Model file for the job. Use its own axes, mm. A direction names the side the tool comes from. Coordinates: 2 decimals unless noted, no trailing zeros. Order: outer loops, then holes, each group sorted by start corner. A loop starts at its lowest first (then second) coordinate and runs counter-clockwise, first axis right, second up. Notation, with made-up numbers: (-24.75, 18) -> (-3.75, 18) arc R20 ccw to (-3.75, 46) -> close; hole circle Ø9 at (-26, -4.75). An arc over 180 degrees is marked (long way). Return JSON: item names as keys, results as strings. Group by question number.
1) Pull direction X, two halves, no side cores. Call faces 3 (the flat face through (-12.8, -40.2, 4.6)), 4 (the flat face through (-75, 51.4, 4.9)), 5 (the flat face through (60, 48.6, 4.9)), 6 (the flat face through (-22, 49, 10)): +X half, -X half, draft (parallel to the pull), parting line (faces both ways), or undercut.
2) Cut at D-D (y = 99.5). Write the cut outline in (x, z).
3) Which spindle directions (+Z, -Z, +X, -X, +Y, -Y) get a long thin tool onto all of the face, cutting with end or side? Do faces 1 (the cylindrical face through (33.763, 135.902, 7.042)), 2 (the flat face through (-7, -50, 5)). Say none if no direction does.
4) Probe line 1 (X direction, y = 65, z = 3.5); line 2 (Y direction, x = 53.25, z = 5); line 3 (Z direction, x = 54.25, y = 125). List the from-to ranges inside material, lowest first.
5) Cut at C-C (z = 1.75). State how many separate pieces and enclosed holes the cut face has, and give its area (3 significant figures).
6) Cut at B-B (x = -30). Write the cut outline in (y, z), and give its area (3 significant figures).
7) Cut at A-A (y = -38). Write the cut outline in (x, z), and give its area (3 significant figures).
8) Flat gauge pin, fed straight in: pin 1 (8.5 mm diameter, centred on x = 30, y = 0, fed in from +Z). Where does the tip first touch, or does it go through?
Autodesk Inventor part; units mm, degrees
ref_plane "Arbeitsebene1" through (-7.5, -50, 10) normal (1, 0, 0) x (0, 0, -1)
ref_plane "YZ Plane" through (0, 0, 0) normal (1, 0, 0) x (0, 1, 0)
ref_plane "XZ Plane" through (0, 0, 0) normal (0, 1, 0) x (-1, 0, 0)
sketch "Skizze1" plane through (0, 0, 0) normal (0, 0, 1) x (1, 0, 0)
  line L0 (-60, 110) -> (60, 110)
  line L1 (60, 110) -> (60, -50)
  line L2 (60, -50) -> (-60, -50)
  line L3 (-60, -50) -> (-60, 110)
  line L4 (-1104, 0) -> (254, 0)
  line L5 (0, -83) -> (0, 148)
  circle A0 centre (-30, 0) radius 2.7
  circle A1 centre (30, 0) radius 2.7
  line L6 (-910, 115) -> (-40, 115)
  point P0 (0, 0)
  dimension "d0" = 110
  dimension "d1" = 120
  dimension "d2" = 60
  dimension "d3" = 5.4
  dimension "d7" = 50
extrude "Extrusion1" add sketch "Skizze1" along normal blind 10 contours L0 L5 L4 A0 L3 | L0 L1 L4 A1 L5 | L4 A0 L5 L2 L3 | L4 A1 L1 L2 L5
sketch "Skizze2" plane through (0, 0, 10) normal (0, 0, 1) x (1, 0, 0)
  line L0 (-60, 110) -> (60, 110)
  line L1 (0, -82) -> (0, 142)
  point P0 (0, 0)
  point P1 (0, 90)
  point P2 (0, 40)
  dimension "d17" = 20
  dimension "d18" = 50
hole "Bohrung2" at (0, 90, 10) at (0, 40, 10) direction (0, 0, -1) diameter 34 end through all
sketch "Skizze5" plane through (0, 0, 10) normal (0, 0, 1) x (1, 0, 0)
  circle A0 centre (30, 0) radius 2.7
  circle A1 centre (-30, 0) radius 2.7
  circle A2 centre (-30, 0) radius 7
  circle A3 centre (30, 0) radius 7
  point P0 (0, 0)
  dimension "d33" = 14
extrude "Extrusion2" cut sketch "Skizze5" against normal blind 6
sketch "Skizze6" plane through (-60, 110, 0) normal (0, 1, 0) x (1, 0, 0)
  line L0 (0, -10) -> (120, -10)
  line L1 (120, 0) -> (120, -10)
  line L2 (0, 0) -> (120, 0)
  line L3 (0, 0) -> (0, -10)
  point P0 (60, 0)
extrude "Extrusion3" add sketch "Skizze6" along normal blind 40
pattern_linear "Rechteckige Anordnung1" count 2 spacing 130 along (0, 1, 0) of "Extrusion2"
sketch "Skizze8" plane through (0, 0, 10) normal (0, 0, 1) x (1, 0, 0)
  circle A0 centre (30, 130) radius 7
  circle A1 centre (-30, 130) radius 7
  point P0 (0, 0)
hole "Bohrung4" at (-30, 130, 10) at (30, 130, 10) direction (0, 0, -1) diameter 5.4 end through all
sketch "Skizze9" plane through (-60, -50, 0) normal (-1, 0, 0) x (0, 0, 1)
  line L0 (10, 0) -> (10, 200)
  line L1 (10, 200) -> (0, 200)
  line L2 (0, 0) -> (0, 200)
  line L3 (0, 0) -> (10, 0)
  point P0 (0, 50)
extrude "Extrusion4" add sketch "Skizze9" along normal blind 15
sketch "Skizze10" plane through (0, 0, 10) normal (0, 0, 1) x (1, 0, 0)
  line L0 (60, 150) -> (-75, 150)
  line L1 (-75, 150) -> (-75, -50)
  line L2 (60, -50) -> (-75, -50)
  line L3 (-75, 120) -> (-28.668, 120)
  line L4 (-53, 93.8234) -> (-53, 98.8806)
  line L5 (60, 150) -> (60, -50)
  line L6 (-75, 10) -> (-27.5048, 10)
  point P0 (0, 0)
  point P1 (-62, 120)
  point P2 (-44, 120)
  point P3 (-62, 10)
  point P4 (-44, 10)
  dimension "d50" = 30
  dimension "d51" = 22
  dimension "d52" = 18
  dimension "d60" = 140
  dimension "d61" = 18
hole "Bohrung6" at (-62, 120, 10) at (-44, 120, 10) at (-62, 10, 10) at (-44, 10, 10) direction (0, 0, -1) diameter 3.242 end through all
sketch "Skizze11" plane through (0, 0, 10) normal (0, 0, 1) x (1, 0, 0)
  circle A0 centre (7.5, -46) radius 1.621
  circle A1 centre (7.5, -30) radius 1.621
  circle A2 centre (-7.5, -30) radius 1.621
  circle A3 centre (-7.5, -46) radius 1.621
  line L0 (-25, -26) -> (25, -26)
  line L1 (-25, -50) -> (-25, -26)
  line L2 (25, -50) -> (-25, -50)
  line L3 (25, -26) -> (25, -50)
  line L4 (-25, -38) -> (25, -38)
  line L5 (-102, 0) -> (87, 0)
  line L6 (0, -90) -> (0, 190)
  circle A4 centre (15, -38) radius 2.067
  circle A5 centre (-15, -38) radius 2.067
  point P0 (0, 0)
  point P1 (-15, -38)
  point P2 (15, -38)
  dimension "d69" = 30
hole "Bohrung7" at (-15, -38, 10) at (15, -38, 10) direction (0, 0, -1) diameter 5.5 end through all counterbore diameter 10 counterbore depth 5.4
sketch "Skizze12" plane through (60, -50, 10) normal (1, 0, 0) x (0, 0, -1)
  line L0 (0, 200) -> (0, 0)
  line L1 (10, 0) -> (0, 0)
  line L2 (10, 200) -> (0, 200)
  line L3 (10, -40) -> (10, 240)
  line L4 (12, 50) -> (-2, 50)
  line L5 (0, 100) -> (10, 100)
  line L6 (5, 200) -> (5, 0)
  point P0 (10, 50)
  point P1 (5, 175)
  point P2 (5, 100)
  point P3 (5, 25)
  dimension "d77" = 25
  dimension "d78" = 25
hole "Bohrung8" at (60, 125, 5) at (60, 50, 5) at (60, -25, 5) direction (-1, 0, 0) diameter 2.459 depth 10 tip angle 118
ref_plane "Arbeitsebene1" through (-7.5, -50, 10) normal (1, 0, 0) x (0, 0, -1)
mirror "Spiegeln1" about plane through (-7.5, -50, 10) normal (1, 0, 0) of "Bohrung8"
hole "Bohrung9" at (8, 65, 10) at (-8, 65, 10) direction (0, 0, -1) diameter 5 end through all
sketch "Skizze13" plane through (0, 0, 10) normal (0, 0, 1) x (1, 0, 0)
  circle A0 centre (-15, 119) radius 2.75
  circle A1 centre (15, 119) radius 2.75
  circle A2 centre (15, 11) radius 2.75
  circle A3 centre (-15, 11) radius 2.75
  point P0 (0, 0)
hole "Bohrung10" at (-15, 11, 10) at (15, 11, 10) at (15, 119, 10) at (-15, 119, 10) direction (0, 0, -1) diameter 4.134 end through all
sketch "Skizze14" plane through (0, 0, 10) normal (0, 0, 1) x (1, 0, 0)
  line L0 (60, 150) -> (60, -50)
  line L1 (60, 150) -> (-75, 150)
  line L2 (-75, 150) -> (-75, -50)
  line L3 (60, -50) -> (-75, -50)
  line L4 (50, 150) -> (50, -50)
  line L5 (-65, 150) -> (-65, -50)
  point P0 (0, 0)
  point P1 (50, 63)
  point P2 (50, 33)
  point P3 (-65, 63)
  point P4 (-65, 33)
  dimension "d101" = 10
  dimension "d102" = 87
  dimension "d103" = 30
  dimension "d104" = 10
hole "Bohrung11" at (50, 63, 10) at (50, 33, 10) at (-65, 63, 10) at (-65, 33, 10) direction (0, 0, -1) diameter 2.459 end through all
properties part number "13_0204_028"
Answers below:
{
 "1": {"face 3": "undercut", "face 4": "-X half", "face 5": "+X half", "face 6": "draft"},
 "2": {"outline": "(-75, 0) -> (-14.1, 0) -> (-14.1, 10) -> (-75, 10) -> close; (14.1, 0) -> (60, 0) -> (60, 10) -> (14.1, 10) -> close"},
 "3": {"face 1": "+Z", "face 2": "+Z, -Z, +X, -X, -Y"},
 "4": {"line 1": "x = -75 to -10.5, -5.5 to 5.5, 10.5 to 60", "line 2": "y = -50 to -26.23, -23.77 to 48.77, 51.23 to 123.77, 126.23 to 150", "line 3": "z = 0 to 3.77, 6.23 to 10"},
 "5": {"separate pieces": "1", "enclosed holes": "22", "area": "24,900 mm^2"},
 "6": {"outline": "(-50, 0) -> (-2.7, 0) -> (-2.7, 4) -> (-7, 4) -> (-7, 10) -> (-50, 10) -> close; (2.7, 0) -> (127.3, 0) -> (127.3, 4) -> (123, 4) -> (123, 10) -> (7, 10) -> (7, 4) -> (2.7, 4) -> close; (132.7, 0) -> (150, 0) -> (150, 10) -> (137, 10) -> (137, 4) -> (132.7, 4) -> close", "area": "1,790 mm^2"},
 "7": {"outline": "(-75, 0) -> (-17.75, 0) -> (-17.75, 4.6) -> (-20, 4.6) -> (-20, 10) -> (-75, 10) -> close; (-12.25, 0) -> (12.25, 0) -> (12.25, 4.6) -> (10, 4.6) -> (10, 10) -> (-10, 10) -> (-10, 4.6) -> (-12.25, 4.6) -> close; (17.75, 0) -> (60, 0) -> (60, 10) -> (20, 10) -> (20, 4.6) -> (17.75, 4.6) -> close", "area": "1,190 mm^2"},
 "8": {"pin 1": "stops at z = 4"}
}
